The model under review builds one solid part; all positions refer to its coordinate system, in mm. Round coordinates to 2 decimals unless told otherwise and drop trailing zeros. Write each loop counter-clockwise with the first axis right and the second up, starting at its lowest first coordinate (ties: lowest second). Pieces come first, ordered by that corner, then holes. Notation, with made-up numbers: (60.5, 29) - (104.5, 29) arc R18 cw to (104.5, 62) - close; hole circle Ø1 at (66, -18.75). An arc over 180 degrees is marked (long way). Return JSON: item names as keys, results as strings.
from build123d import *

# Parameters (mm, degrees)
BOSS_EXTRUDE1_DEPTH = 80
BOSS_EXTRUDE2_START = -74
SKETCH2_R           = 2.5
BOSS_EXTRUDE2_DEPTH = 74
SKETCH3_R           = 2.5
CUT_EXTRUDE1_DEPTH  = 6
SKETCH4_R           = 2.5
CUT_EXTRUDE2_DEPTH  = 6
CUT_EXTRUDE3_DEPTH  = 12
CUT_EXTRUDE4_START  = -6
SKETCH6_R           = 2.5
CUT_EXTRUDE4_DEPTH  = 6


with BuildPart() as part:
    # Sketch1 → Boss-Extrude1 (new body)
    with BuildSketch(Plane.XY):
        with BuildLine():
            Line((0, 25.5), (0, 28.45))
            Line((0, 28.45), (-5, 28.9))
            Line((-5, 28.9), (-5, -28.9))
            Line((-5, -28.9), (0, -28.45))
            Line((0, -28.45), (0, -25.5))
            ThreePointArc((0, -25.5), (-2.5, -23), (0, -20.5))
            Line((0, -20.5), (0, 20.5))
            ThreePointArc((0, 20.5), (-2.5, 23), (0, 25.5))
        make_face()
        with BuildLine():
            Line((5, 28), (0, 28.45))
            Line((0, 28.45), (0, 25.5))
            ThreePointArc((0, 25.5), (1.767766953, 24.767766953), (2.5, 23))
            ThreePointArc((2.5, 23), (1.767766953, 21.232233047), (0, 20.5))
            Line((0, 20.5), (0, -20.5))
            ThreePointArc((0, -20.5), (1.767766953, -21.232233047), (2.5, -23))
            ThreePointArc((2.5, -23), (1.767766953, -24.767766953), (0, -25.5))
            Line((0, -25.5), (0, -28.45))
            Line((0, -28.45), (5, -28))
            Line((5, -28), (5, 28))
        make_face()
    extrude(amount=BOSS_EXTRUDE1_DEPTH)

    # Sketch2 → Boss-Extrude2 (add)
    with BuildSketch(Plane.XY.offset(80).offset(BOSS_EXTRUDE2_START)):
        with Locations((0, 23)):
            Circle(SKETCH2_R)
        with Locations((0, -23)):
            Circle(SKETCH2_R)
    extrude(amount=BOSS_EXTRUDE2_DEPTH)

    # Sketch3 → Cut-Extrude1 (cut)
    with BuildSketch(Plane.XY.offset(80)):
        with Locations((0, 23.038742356)):
            Circle(SKETCH3_R)
    extrude(amount=-CUT_EXTRUDE1_DEPTH, mode=Mode.SUBTRACT)

    # Sketch4 → Cut-Extrude2 (cut)
    with BuildSketch(Plane.XY.offset(80)):
        with Locations((0, -23.038742356)):
            Circle(SKETCH4_R)
    extrude(amount=-CUT_EXTRUDE2_DEPTH, mode=Mode.SUBTRACT)

    # Sketch5 → Cut-Extrude3 (cut)
    with BuildSketch(Plane.XY.offset(80)):
        Polygon((-5, 28.9), (5, 28), (5, -28), (-5, -28.9), align=None)
    extrude(amount=-CUT_EXTRUDE3_DEPTH, mode=Mode.SUBTRACT)

    # Sketch6 → Cut-Extrude4 (cut)
    with BuildSketch(Plane.XY.offset(68).offset(CUT_EXTRUDE4_START)):
        with Locations((0, 23)):
            Circle(SKETCH6_R)
        with Locations((0, -23)):
            Circle(SKETCH6_R)
    extrude(amount=CUT_EXTRUDE4_DEPTH, mode=Mode.SUBTRACT)


solid = part.part
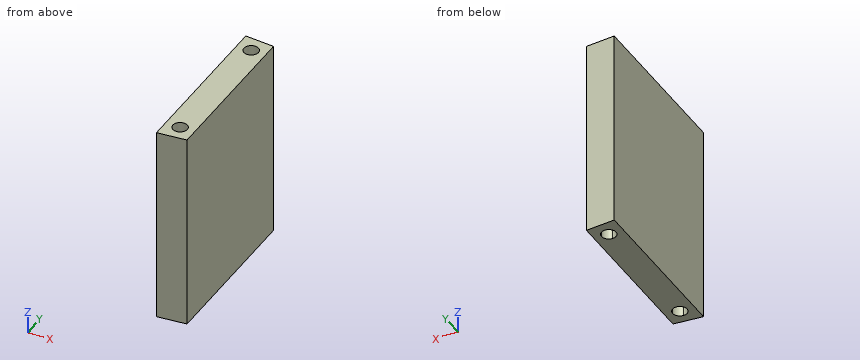
(1) Clearance check with a flat-ended pin moving along its axis: pin 1 Ø4 at (x, y) = (0, 23) entering from -Z. State where the tip first meets the part, or that it passes through.
Filled in:
{"pin 1": "stops at z = 6"}
(2) Add section C-C (x = 4). Write out the cut boundary in (y, z), plus the area to 3 significant figures.
Filled in:
{"outline": "(-28.09, 0) - (28.09, 0) - (28.09, 68) - (-28.09, 68) - close", "area": "3,820 mm2"}
(3) Add section A-A (x = -0.75). Write out the cut boundary in (y, z).
Filled in:
{"outline": "(-28.52, 0) - (-25.38, 0) - (-25.38, 6) - (-20.62, 6) - (-20.62, 0) - (20.62, 0) - (20.62, 6) - (25.38, 6) - (25.38, 0) - (28.52, 0) - (28.52, 68) - (25.38, 68) - (25.38, 62) - (20.62, 62) - (20.62, 68) - (-20.62, 68) - (-20.62, 62) - (-25.38, 62) - (-25.38, 68) - (-28.52, 68) - close"}
(4) Add section B-B (z = 34.5). Write out the cut boundary in (x, y), plus the area to 3 significant figures.
Filled in:
{"outline": "(-5, -28.9) - (5, -28) - (5, 28) - (-5, 28.9) - close", "area": "569 mm2"}
(5) Wall thickness on line 1 (Y direction, x = 0, z = 63.8); line 2 (Z direction, x = 2, y = -22); line 3 (Y direction, x = -1.25, z = 7): over which ranges is each line inside the solid? List them lowest first.
Filled in:
{"line 1": "y = -28.45 to -25.5, -20.5 to 20.5, 25.5 to 28.45", "line 2": "z = 6 to 62", "line 3": "y = -28.56 to 28.56"}
